The listing builds one solid part. Answer for the finished solid, in the listing's coordinates (mm). A direction names the side the tool comes from. Coordinates: 2 decimals unless noted, no trailing zeros. Order: outer loops, then holes, each group sorted by start corner. A loop starts at its lowest first (then second) coordinate and runs counter-clockwise, first axis right, second up. Notation, with made-up numbers: (1, -32.75) -> (54, -32.75) arc R10 cw to (54, -28.75) -> close; hole circle Ø6 at (58, 79.5). An arc over 180 degrees is marked (long way). Answer in a Markdown table with one row per item. Add a question column.
```python
from build123d import *

# Parameters (mm, degrees)
F1_DEPTH      = 800
F3_DEPTH      = 200
F4_W          = 25
F4_H          = 120
F5_DEPTH      = 130
F6_W          = 15
F6_H          = 60
F7_DEPTH      = 60
F8_R          = 7.5
F9_DEPTH      = 65
F9_DEPTH_BACK = 5
F10_R         = 17.5
F11_DEPTH     = 160.001


with BuildPart() as f1:
    # F0 (on Front) → F1 (new body)
    with BuildSketch(Plane.XZ):
        Polygon((0, 100), (0, 0), (10, 0), (10, 90), (170, 90), (170, 0), (180, 0), (180, 100), align=None)
    extrude(amount=F1_DEPTH)

    # F2 (on face) → F3 (join)
    with BuildSketch(Plane.XY.offset(100)):
        Polygon((10, 0), (0, 0), (0, -100), (180, -100), (180, 0), (170, 0), (170, -90), (10, -90), align=None)
    extrude(amount=F3_DEPTH)

    # F4 (on face) → F5 (join)
    with BuildSketch(Plane.XY.offset(100)):
        with Locations((32.5, -440)):
            Rectangle(F4_W, F4_H)
        with Locations((147.5, -440)):
            Rectangle(F4_W, F4_H)
    extrude(amount=F5_DEPTH)

    # F6 (on face) → F7 (join)
    with BuildSketch(Plane.XZ.offset(100)):
        with Locations((67.5, 165)):
            Rectangle(F6_W, F6_H)
        with Locations((112.5, 165)):
            Rectangle(F6_W, F6_H)
    extrude(amount=F7_DEPTH)

    # F8 (on face) → F9 (join, two sides)
    with BuildSketch(Plane(origin=(60, 0, 0), x_dir=(0, -1, 0), z_dir=(-1, 0, 0))) as f9_sk:
        with Locations((140, 165)):
            Circle(F8_R)
    extrude(amount=-F9_DEPTH)
    extrude(f9_sk.sketch, amount=F9_DEPTH_BACK)

    # F10 (on face) → F11 (cut, through all)
    with BuildSketch(Plane(origin=(20, 0, 0), x_dir=(0, -1, 0), z_dir=(-1, 0, 0))):
        with Locations((440, 165)):
            Circle(F10_R)
    extrude(amount=-F11_DEPTH, mode=Mode.SUBTRACT)


solid = f1.part
```
Q1. A cutting plane is placed at A-A (x = 89.5). Determine the outline of the cut face in (y, z), then the cut area to 3 significant figures.
Q2. A cutting plane is placed at B-B (y = -140). Determine the outline of the cut face in (x, z), then the cut area to 3 significant figures.
Q3. A cutting plane is placed at C-C (z = 213). Determine the outline of the cut face in (x, y).
Q4. Straight lines are drawn through the part: line 1 (Z direction, x = 25.75, y = -440); line 2 (X direction, y = -32.5, z = 79); line 3 (Y direction, x = 27, z = 198). For each, find the intervals that lie inside material, in ascending order.
Q5. Determine the mould class of faces 1 (the face through (20, -454, 150)), 2 (the face through (91, -44, 100)), 3 (the face through (67, -130, 195)) for opening direction X: +X half, -X half, draft (parallel to the pull), parting line (faces both ways), or undercut.
Q6. For faces 4 (the face through (10, -46, 199)), 5 (the face through (147, -380, 164)), 6 (the face through (45, -454, 150)), 7 (the face through (32, -500, 164)), 8 (the face through (67, -130, 135)), determine the directions among +Z, -Z, +X, -X, +Y, -Y from which every point of the face is accessible in a straight line to the end or side of a thin tool.
Q7. Given pin 1 (3 mm diameter, centred on x = 48.5, z = 188.5, fed in from -Y); pin 2 (3 mm diameter, centred on x = 153.5, y = -598, fed in from -Z); pin 3 (4 mm diameter, centred on x = 125.5, z = 156.5, fed in from +Y); pin 4 (10 mm diameter, centred on y = -550.5, z = 79.5, fed in from -X), each flat-ended and moving along its own axis, determine where each tip first touches the part or whether it passes through.
Q8. A cutting plane is placed at D-D (x = 145). Determine the outline of the cut face in (y, z), then the cut area to 3 significant figures.
Returned:
| question | item | result |
|---|---|---|
| 1 | outline | (-800, 90) -> (0, 90) -> (0, 100) -> (-90, 100) -> (-90, 300) -> (-100, 300) -> (-100, 100) -> (-800, 100) -> close; circle Ø15 at (-140, 165) |
| 1 | area | 10,200 mm² |
| 2 | outline | (0, 0) -> (10, 0) -> (10, 90) -> (170, 90) -> (170, 0) -> (180, 0) -> (180, 100) -> (0, 100) -> close; (55, 157.5) -> (60, 157.5) -> (60, 135) -> (75, 135) -> (75, 157.5) -> (105, 157.5) -> (105, 135) -> (120, 135) -> (120, 157.5) -> (125, 157.5) -> (125, 172.5) -> (120, 172.5) -> (120, 195) -> (105, 195) -> (105, 172.5) -> (75, 172.5) -> (75, 195) -> (60, 195) -> (60, 172.5) -> (55, 172.5) -> close |
| 2 | area | 6,000 mm² |
| 3 | outline | (0, -100) -> (180, -100) -> (180, 0) -> (170, 0) -> (170, -90) -> (10, -90) -> (10, 0) -> (0, 0) -> close; (20, -500) -> (45, -500) -> (45, -380) -> (20, -380) -> close; (135, -500) -> (160, -500) -> (160, -380) -> (135, -380) -> close |
| 4 | line 1 | z = 90 to 147.5, 182.5 to 230 |
| 4 | line 2 | x = 0 to 10, 170 to 180 |
| 4 | line 3 | y = -500 to -380, -100 to -90 |
| 5 | face 1 | -X half |
| 5 | face 2 | undercut |
| 5 | face 3 | draft |
| 6 | face 4 | +Z, +Y |
| 6 | face 5 | +Z, +X, -X |
| 6 | face 6 | +Z, -Y |
| 6 | face 7 | +Z, +X, -X, -Y |
| 6 | face 8 | +X, -X, -Y |
| 7 | pin 1 | stops at y = -100 |
| 7 | pin 2 | stops at z = 90 |
| 7 | pin 3 | stops at y = -90 |
| 7 | pin 4 | stops at x = 0 |
| 8 | outline | (-800, 90) -> (0, 90) -> (0, 100) -> (-90, 100) -> (-90, 300) -> (-100, 300) -> (-100, 100) -> (-380, 100) -> (-380, 230) -> (-500, 230) -> (-500, 100) -> (-800, 100) -> close; hole circle Ø35 at (-440, 165) |
| 8 | area | 24,600 mm² |
